Can you work these out from the model? Positions are in its coordinate system, mm. A direction names the side the tool comes from. Round coordinates to 2 decimals unless told otherwise and drop trailing zeros. Loops run counter-clockwise (first coordinate to the right, second up) from the corner with the lowest first, then second, coordinate; pieces in that order, holes last. Notation, with made-up numbers: (62, 27) - (82, 27) arc R12 cw to (82, 32) - close; hole circle Ø7 at (73, 77.25). An arc over 180 degrees is marked (long way). Answer as CSV lines item,"result".
```python
from build123d import *

# Parameters (mm, degrees)
F0_W     = 25.099074
F0_H     = 25.4
F1_DEPTH = 152.4
F2_W     = 19.695762
F2_H     = 19.05
F3_DEPTH = 203.2
F4_R     = 3.175
F5_DEPTH = 25.4
F6_W     = 19.695762
F6_H     = 3.175
F7_DEPTH = 203.2
F8_R     = 3.175
F9_DEPTH = 25.100073


with BuildPart() as f1:
    # F0 (on Front) → F1 (new body)
    with BuildSketch(Plane.XZ):
        Rectangle(F0_W, F0_H)
    extrude(amount=F1_DEPTH)

    # F2 (on face) → F3 (cut)
    with BuildSketch(Plane.XZ.offset(152.4)):
        Rectangle(F2_W, F2_H)
    extrude(amount=-F3_DEPTH, mode=Mode.SUBTRACT)

    # F4 (on face) → F5 (cut)
    with BuildSketch(Plane.YZ.offset(12.549537)):
        with Locations((-139.7, 0)):
            Circle(F4_R)
    extrude(amount=-F5_DEPTH, mode=Mode.SUBTRACT)

    # F6 (on face) → F7 (cut)
    with BuildSketch(Plane(origin=(0, 0, 0), x_dir=(-1, 0, 0), z_dir=(0, 1, 0))):
        with Locations((0, 11.1125)):
            Rectangle(F6_W, F6_H)
    extrude(amount=-F7_DEPTH, mode=Mode.SUBTRACT)

    # F8 (on face) → F9 (cut, through all)
    with BuildSketch(Plane.YZ.offset(12.549537)):
        with Locations((-12.7, 0)):
            Circle(F8_R)
        with BuildLine():
            add(Edge.make_bspline(
                [(-60.325, 0), (-60.325, 5.499261), (-74.6125, 2.749631), (-88.9, 0), (-74.6125, -2.749631), (-60.325, -5.499261), (-60.325, 0)],
                knots=[0, 0, 0, 2.094395, 2.094395, 4.18879, 4.18879, 6.283185, 6.283185, 6.283185], degree=2, weights=[1, 0.5, 1, 0.5, 1, 0.5, 1]))
        make_face()
        with BuildLine():
            add(Edge.make_bspline(
                [(-28.575, 0), (-28.575, 5.499261), (-42.8625, 2.749631), (-57.15, 0), (-42.8625, -2.749631), (-28.575, -5.499261), (-28.575, 0)],
                knots=[0, 0, 0, 2.094395, 2.094395, 4.18879, 4.18879, 6.283185, 6.283185, 6.283185], degree=2, weights=[1, 0.5, 1, 0.5, 1, 0.5, 1]))
        make_face()
    extrude(amount=-F9_DEPTH, mode=Mode.SUBTRACT)


solid = f1.part
```
Q1. I'm going to push flat-ended pins straight in: pin 1 Ø1 at (x, y) = (-3.5, -18.5) entering from +Z (3 decimals); pin 2 Ø4 at (y, z) = (-12.7, 0) entering from +X. Where does each tip first touch, or does it pass through?
Checks:
pin 1,"z = -9.525"
pin 2,"through"
Q2. Imagine slicing it at A-A (z = -5.25). Write out the boundary of the cut face in (x, y), then the cut area to 3 significant figures.
Checks:
outline,"(-12.55, -152.4) - (-9.85, -152.4) - (-9.85, 0) - (-12.55, 0) - close; (9.85, -152.4) - (12.55, -152.4) - (12.55, 0) - (9.85, 0) - close"
area,"823 mm²"
Q3. On a 3-axis mill with a long thin cutter (end or side, diameter ignored), from which of +Z, -Z, +X, -X, +Y, -Y can I reach the whole of each face in a straight line? I mean faces 4 (the flat face through (0, -77, -9.525)), 5 (the cylindrical face through (11.22, -136.77, -1.22)). Say none if no direction works.
Checks:
face 4,"+Z, +Y, -Y"
face 5,"+X, -X"
Q4. Imagine slicing it at D-D (x = -1.75). Write out the boundary of the cut face in (y, z) (3 decimals), then the cut area to 3 significant figures.
Checks:
outline,"(-152.4, -12.7) - (0, -12.7) - (0, -9.525) - (-152.4, -9.525) - close"
area,"484 mm²"
Q5. If I drill on line 1 along X through (y, z) = (-101, -1.75); line 2 along Z through (x, y) = (-11.35, -139.7) (3 decimals); line 3 along Z through (x, y) = (-4.5, -132) (3 decimals), over which ranges is the centre line in solid material (lowest first)? Write a range as [from, to].
Checks:
line 1,"[-12.55, -9.85], [9.85, 12.55]"
line 2,"[-12.7, -3.175], [3.175, 12.7]"
line 3,"[-12.7, -9.525]"
Q6. Imagine slicing it at C-C (y = -83). Write out the boundary of the cut face in (x, z) (3 decimals).
Checks:
outline,"(-12.55, -12.7) - (12.55, -12.7) - (12.55, 12.7) - (9.848, 12.7) - (9.848, -9.525) - (-9.848, -9.525) - (-9.848, 12.7) - (-12.55, 12.7) - close"
Q7. We'd pull the mould along Z, two halves only. Please class faces 1 (the flat face through (0, -75, -12.7)), 2 (the cylindrical face through (11.22, -9.67, 0.95)), 3 (the flat face through (-9.848, -75, 4)): pulls with the +Z half, pulls with the -Z half, needs draft (parallel to the pull), parting line crosses it, or undercut.
Checks:
face 1,"pulls with the -Z half"
face 2,"undercut"
face 3,"needs draft"
Q8. Imagine slicing it at B-B (y = -139.7). Write out the boundary of the cut face in (x, z) (3 decimals).
Checks:
outline,"(-12.55, -12.7) - (12.55, -12.7) - (12.55, -3.175) - (9.848, -3.175) - (9.848, -9.525) - (-9.848, -9.525) - (-9.848, -3.175) - (-12.55, -3.175) - close; (-12.55, 3.175) - (-9.848, 3.175) - (-9.848, 12.7) - (-12.55, 12.7) - close; (9.848, 3.175) - (12.55, 3.175) - (12.55, 12.7) - (9.848, 12.7) - close"
